CAD build for the part. Positions are in the model's coordinates, mm. Round coordinates to 2 decimals unless told otherwise and drop trailing zeros. Loops run counter-clockwise (first coordinate to the right, second up) from the corner with the lowest first, then second, coordinate; pieces in that order, holes last. Notation, with made-up numbers: (82.5, 81.25) - (112.5, 81.25) arc R21 ccw to (112.5, 102.25) - close; hole circle Ø5 at (69.5, -33.5). An arc over 180 degrees is marked (long way). Use one line per item in the form item = value.
from build123d import *

# Parameters (mm, degrees)
SKETCH1_W           = 38.1
SKETCH1_H           = 57.15
SKETCH1_R           = 2.5527
BOSS_EXTRUDE1_DEPTH = 3.175
FILLET1_R           = 2.54


with BuildPart() as part:
    # Sketch1 → Boss-Extrude1 (new body)
    with BuildSketch(Plane.XY):
        Rectangle(SKETCH1_W, SKETCH1_H)
        with Locations((-9.525, 3.175)):
            Circle(SKETCH1_R, mode=Mode.SUBTRACT)
        with Locations((-9.525, 19.05)):
            Circle(SKETCH1_R, mode=Mode.SUBTRACT)
        with Locations((9.525, 3.175)):
            Circle(SKETCH1_R, mode=Mode.SUBTRACT)
        with Locations((9.525, 19.05)):
            Circle(SKETCH1_R, mode=Mode.SUBTRACT)
        with Locations((-9.525, -9.525)):
            Circle(SKETCH1_R, mode=Mode.SUBTRACT)
        with Locations((9.525, -9.525)):
            Circle(SKETCH1_R, mode=Mode.SUBTRACT)
        with Locations((-9.525, -22.225)):
            Circle(SKETCH1_R, mode=Mode.SUBTRACT)
        with Locations((9.525, -22.225)):
            Circle(SKETCH1_R, mode=Mode.SUBTRACT)
    extrude(amount=BOSS_EXTRUDE1_DEPTH)

    # Fillet1
    fillet1_edges = [part.edges().sort_by_distance(p)[0] for p in [
        (19.05, -28.575, 1.5875),
        (-19.05, -28.575, 1.5875),
        (-19.05, 28.575, 1.5875),
        (19.05, 28.575, 1.5875),
    ]]
    fillet(fillet1_edges, radius=FILLET1_R)


solid = part.part
1) Slice it at B-B (z = 1.75). State how many separate pieces and enclosed holes the cut face has, plus the area to 3 significant figures.
Report:
separate_pieces = 1
enclosed_holes = 8
area = 2,010 mm^2
2) Flat gauge pin, fed straight in: pin 1 (3 mm diameter, centred on x = 9.525, y = 19.05, fed in from +Z). Where does the tip first touch, or does it go through?
Report:
pin_1 = through
3) Drill centre lines: probe 1 along X at (y, z) = (-9, 1.5); probe 2 along X at (y, z) = (-24, 1.5); probe 3 along Y at (x, z) = (9, 3) (3 decimals). Where is each one in solid material? Low to high.
Report:
probe_1 = -19.05 to -12.02, -7.03 to 7.03, 12.02 to 19.05
probe_2 = -19.05 to -11.36, -7.69 to 7.69, 11.36 to 19.05
probe_3 = -28.575 to -24.723, -19.727 to -12.023, -7.027 to 0.677, 5.673 to 16.552, 21.548 to 28.575
4) Two-plate mould, pull along X, no slides. Class faces 1 (the cylindrical face through (-18.326, -27.811, 1.61)), 2 (the cylindrical face through (7.5, 1.62, 1.57)), 3 (the flat face through (0, 28.575, 2)): +X half, -X half, draft (parallel to the pull), parting line (faces both ways), or undercut.
Report:
face_1 = -X half
face_2 = undercut
face_3 = draft
5) Slice it at A-A (y = 19.05). Write the cut outline in (x, z) (3 decimals), plus the area to 3 significant figures.
Report:
outline = (-19.05, 0) - (-12.078, 0) - (-12.078, 3.175) - (-19.05, 3.175) - close; (-6.972, 0) - (6.972, 0) - (6.972, 3.175) - (-6.972, 3.175) - close; (12.078, 0) - (19.05, 0) - (19.05, 3.175) - (12.078, 3.175) - close
area = 88.5 mm^2
